```python
from build123d import *

# Parameters (mm, degrees)
F0_R     = 6
F1_DEPTH = 22
F2_DEPTH = 24.7


# Not quite as in the source:
# - the dataset's text gives a spline's control points without its knots; the knots are read off the source's solid
# - a feature names something its author has since deleted; it is built from what else it names


with BuildPart() as f1:
    # F0 (on Top) → F1 (new body)
    with BuildSketch(Plane.XY):
        with BuildLine():
            ThreePointArc((-44.2506901264, 54.2390673163), (-37.2170072256, 49.3508335883), (-28.7157507853, 50.3978116504))
            ThreePointArc((-28.7157507853, 50.3978116504), (-24.0543074262, 54.8133136372), (-22.3365694268, 61))
            ThreePointArc((-22.3365694268, 61), (-28.149883064, 71.2822620006), (-39.9573880683, 71.6021883496))
            ThreePointArc((-39.9573880683, 71.6021883496), (-45.9857358385, 63.8804377989), (-44.2506901264, 54.2390673163))
        make_face()
        with Locations((-34.3365694268, 61)):
            Circle(F0_R, mode=Mode.SUBTRACT)
        with BuildLine():
            ThreePointArc((-41.1910181988, -70.8496970528), (-28.7801940464, -71.6361032635), (-22.3365694268, -61))
            ThreePointArc((-22.3365694268, -61), (-39.8929448072, -50.3638967365), (-41.1910181988, -70.8496970528))
        make_face()
        with Locations((-34.3365694268, -61)):
            Circle(F0_R, mode=Mode.SUBTRACT)
        with BuildLine():
            ThreePointArc((-18.536827307, 82.9584370096), (-23.5181968435, 66.7354296949), (-7.2951893768, 61.7540606536))
            ThreePointArc((-7.2951893768, 61.7540606536), (-2.6337464761, 66.1695626111), (-0.9160086655, 72.35624866))
            ThreePointArc((-0.9160086655, 72.35624866), (-6.7293223028, 82.6385106606), (-18.536827307, 82.9584370096))
        make_face()
        with Locations((-12.9160086655, 72.35624866)):
            Circle(F0_R, mode=Mode.SUBTRACT)
        with BuildLine():
            Line((-22.3365694268, 51.1162809556), (-22.3365694268, -27.5282078784))
            add(Edge.make_bspline(
                [(-19.1679852382, 55.4596212318), (-19.1490913177, 55.4067702681), (-18.2627780559, 52.9264771043), (-16.5142433132, 47.9330355336), (-14.0597955985, 40.2848666723), (-11.8817933237, 32.380636116), (-10.1403594344, 24.1713941631), (-9.0428174028, 15.5795000988), (-8.9070069048, 8.0286707772), (-9.4009784523, 2.5365834769), (-9.8823537024, -0.64961691), (-10.3506440426, -3.0593767725), (-10.9326328555, -5.4817632435), (-11.6386397696, -7.9166705081), (-12.4443293031, -10.2769526895), (-13.6414482379, -13.3297795407), (-15.3453349713, -16.9551929086), (-17.6521060756, -20.9929507786), (-20.005676914, -24.5007883382), (-21.6047261121, -26.6086284401), (-22.3365694268, -27.5282078784)],
                knots=[0.0611387127, 0.0611387127, 0.0611387127, 0.0611387127, 0.0625, 0.125, 0.1875, 0.25, 0.3125, 0.375, 0.4375, 0.46875, 0.484375, 0.5, 0.515625, 0.53125, 0.546875, 0.5625, 0.59375, 0.625, 0.65625, 0.6818147445, 0.6818147445, 0.6818147445, 0.6818147445], degree=3))
            Line((-19.1679852382, 55.4596212318), (-21.0545147962, 54.4594654001))
            ThreePointArc((-21.0545147962, 54.4594654001), (-22.0050663394, 52.9065704787), (-22.3365694268, 51.1162809556))
        make_face()
        with BuildLine():
            ThreePointArc((-41.1910181988, -70.8496970528), (-39.8929448072, -50.3638967365), (-22.3365694268, -61))
            Line((-22.3365694268, -61), (-22.3365694268, -27.5282078784))
            Line((-22.3365694268, -27.5282078784), (-22.3365694268, 51.1162809556))
            ThreePointArc((-22.3365694268, 51.1162809556), (-22.0050663394, 52.9065704787), (-21.0545147962, 54.4594654001))
            Line((-21.0545147962, 54.4594654001), (-28.7157507853, 50.3978116504))
            ThreePointArc((-28.7157507853, 50.3978116504), (-37.2170072256, 49.3508335883), (-44.2506901264, 54.2390673163))
            add(Edge.make_bspline(
                [(-44.2506901264, 54.2390673163), (-37.1132332482, 34.6511342855), (-23.4734527351, -2.7816813244), (-51.824990918, -23.6902906337), (-65.3406685812, -33.657792996)],
                knots=[0, 0, 0, 0, 0.523282385, 1, 1, 1, 1], degree=3))
            ThreePointArc((-65.3406685812, -33.657792996), (-53.1694343986, -33.3492849771), (-46.993012785, -43.8414694388))
            ThreePointArc((-46.993012785, -43.8414694388), (-53.4366374046, -54.4775727023), (-65.847461557, -53.6911664916))
            Line((-65.847461557, -53.6911664916), (-41.1910181988, -70.8496970528))
        make_face()
        with BuildLine():
            Line((-21.0545147962, 54.4594654001), (-19.1679852382, 55.4596212318))
            Line((-19.1679852382, 55.4596212318), (-7.2951893768, 61.7540606536))
            ThreePointArc((-7.2951893768, 61.7540606536), (-23.5181968435, 66.7354296949), (-18.536827307, 82.9584370096))
            Line((-18.536827307, 82.9584370096), (-39.9573880683, 71.6021883496))
            ThreePointArc((-39.9573880683, 71.6021883496), (-28.149883064, 71.2822620006), (-22.3365694268, 61))
            ThreePointArc((-22.3365694268, 61), (-24.0543074262, 54.8133136372), (-28.7157507853, 50.3978116504))
            Line((-28.7157507853, 50.3978116504), (-21.0545147962, 54.4594654001))
        make_face()
    extrude(amount=F1_DEPTH)

    # F0 (on Top) → F2 (join)
    with BuildSketch(Plane.XY):
        with BuildLine():
            ThreePointArc((-70.6743202458, -41.0942788729), (-70.1985453114, -48.1351905289), (-65.847461557, -53.6911664916))
            ThreePointArc((-65.847461557, -53.6911664916), (-53.4366374046, -54.4775727023), (-46.993012785, -43.8414694388))
            ThreePointArc((-46.993012785, -43.8414694388), (-53.1694343986, -33.3492849771), (-65.3406685812, -33.657792996))
            ThreePointArc((-65.3406685812, -33.657792996), (-68.7442285851, -36.8476299769), (-70.6743202458, -41.0942788729))
        make_face()
        with Locations((-58.993012785, -43.8414694388)):
            Circle(F0_R, mode=Mode.SUBTRACT)
    extrude(amount=F2_DEPTH)


solid = f1.part
```
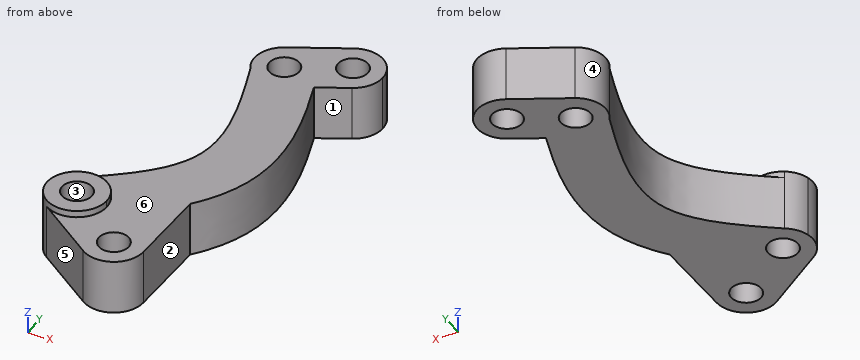
Input: part model. Units: mm. Frame: model coordinates. Face numbers are marked on the shaded views. A direction names the side the tool comes from. Coordinates: 2 decimals unless noted, no trailing zeros. Loops run counter-clockwise (first coordinate to the right, second up) from the corner with the lowest first, then second, coordinate; pieces in that order, holes last.
Q1. Section D-D, the plane x = -25. Return the cut outline in (y, z).
Results are:
outline: (-68.54, 0) - (79.53, 0) - (79.53, 22) - (-68.54, 22) - close
Q2. Contact query for flat-ended pins moving along their axis: pin 1 (19 mm diameter, centred on x = -34.34, y = 61, fed in from +Z); pin 2 (8 mm diameter, centred on x = -58.5, y = -43.5, fed in from +Z); pin 3 (2 mm diameter, centred on y = -21.5, z = 16, fed in from +X); pin 4 (12 mm diameter, centred on y = 48.5, z = 5, fed in from +X). Output: stop coordinate, or through.
Results are:
pin 1: stops at z = 22
pin 2: passes through
pin 3: stops at x = -17.41
pin 4: stops at x = -14.79
Q3. Section A-A, the plane x = -38.5. Give the number of separate pieces and of enclosed holes in the cut face, and give its area (3 significant figures).
Results are:
separate pieces: 4
enclosed holes: 0
area: 1,770 mm2
Q4. Mould query, pull axis Y, two halves, no side actions, for the marked faces 4, 5 and 6. Classes: +Y half, -Y half, draft (parallel to the pull), parting line (faces both ways), or undercut.
Results are:
face 4: undercut
face 5: -Y half
face 6: draft
Q5. Line query: line 1 along Z through (x, y) = (-15, 17.5); line 2 along X through (y, z) = (75.5, 18); line 3 along X through (y, z) = (-63.5, 6.75). Output: solid intervals per line, ascending.
Results are:
line 1: z = 0 to 22
line 2: x = -32.61 to -18.03, -7.81 to -1.34
line 3: x = -51.75 to -39.79, -28.88 to -22.6
Q6. Set-up query: the marked faces 1, 2 and 3. Return all of +Z, -Z, +X, -X, +Y, -Y with unobstructed straight access to the full face (end or side cutting, diameter ignored); none if empty.
Results are:
face 1: +Z, -Z, +X
face 2: +Z, -Z, +X, -Y
face 3: +Z, -Z
